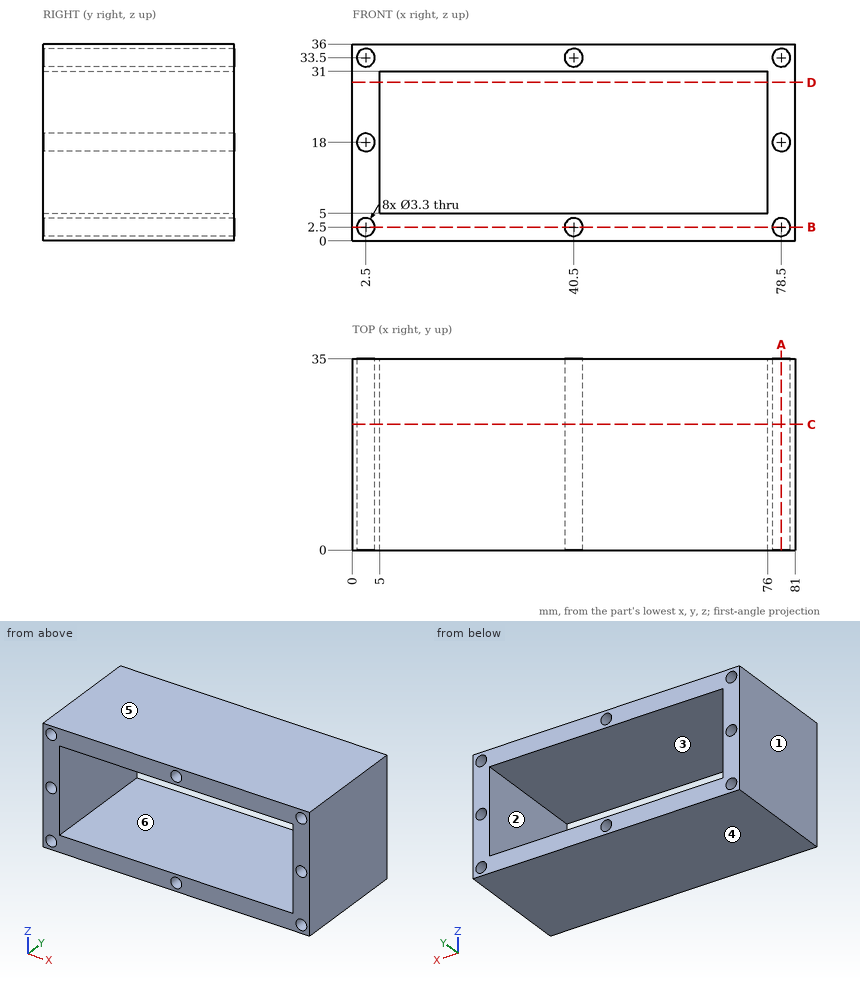
Geometry: see drawing. Coordinates: mm, zero at the bounding-box minimum. A direction names the side the tool comes from. Coordinates: 2 decimals unless noted, no trailing zeros. Loops run counter-clockwise (first coordinate to the right, second up) from the corner with the lowest first, then second, coordinate; pieces in that order, holes last. Notation, with made-up numbers: (18.25, 62.5) -> (27.25, 62.5) arc R22 cw to (27.25, 81.5) -> close; hole circle Ø8 at (-14, -22.75). An arc over 180 degrees is marked (long way). Write item = value, one per line. Start each with the question number.
Item 1: Reachability of the marked faces 5 and 6 from +Z, -Z, +X, -X, +Y, -Y: full face, straight path, thin tool, end or side. Return the list, or none.
Item 2: Material intervals for line 1 (Z direction, x = 21.5, y = 6); line 2 (X direction, y = 30, z = 29.5); line 3 (X direction, y = 27.5, z = 17.5), sorted ascending.
Item 3: Cut plane D-D, the plane z = 29. Return loops of the section in (x, y), plus the area to 3 significant figures.
Item 4: Mould query, pull axis X, two halves, no side actions, for the marked faces 1, 2, 3 and 4. Classes: pulls with the +X half, pulls with the -X half, needs draft (parallel to the pull), parting line crosses it, or undercut.
Item 5: Cut plane B-B, the plane z = 2.5. Return loops of the section in (x, y), plus the area to 3 significant figures.
Item 6: Cut plane C-C, the plane y = 23. Count the separate pieces of the cut face and the enclosed holes in it, plus the area to 3 significant figures.
Item 7: Cut plane A-A, the plane x = 78.5. Return loops of the section in (y, z), plus the area to 4 significant figures.
Ans:
q1.face_5 = +Z, +X, -X, +Y, -Y
q1.face_6 = +Y, -Y
q2.line_1 = 0 to 5, 31 to 36
q2.line_2 = 0 to 5, 76 to 81
q2.line_3 = 0 to 0.93, 4.07 to 5, 76 to 76.93, 80.07 to 81
q3.outline = (0, 0) -> (5, 0) -> (5, 35) -> (0, 35) -> close; (76, 0) -> (81, 0) -> (81, 35) -> (76, 35) -> close
q3.area = 350 mm²
q4.face_1 = pulls with the -X half
q4.face_2 = undercut
q4.face_3 = undercut
q4.face_4 = needs draft
q5.outline = (0, 0) -> (0.85, 0) -> (0.85, 35) -> (0, 35) -> close; (4.15, 0) -> (38.85, 0) -> (38.85, 35) -> (4.15, 35) -> close; (42.15, 0) -> (76.85, 0) -> (76.85, 35) -> (42.15, 35) -> close; (80.15, 0) -> (81, 0) -> (81, 35) -> (80.15, 35) -> close
q5.area = 2,490 mm²
q6.separate_pieces = 1
q6.enclosed_holes = 9
q6.area = 1,000 mm²
q7.outline = (0, 0) -> (35, 0) -> (35, 0.85) -> (0, 0.85) -> close; (0, 4.15) -> (35, 4.15) -> (35, 16.35) -> (0, 16.35) -> close; (0, 19.65) -> (35, 19.65) -> (35, 31.85) -> (0, 31.85) -> close; (0, 35.15) -> (35, 35.15) -> (35, 36) -> (0, 36) -> close
q7.area = 913.5 mm²
